```python
from build123d import *

# Parameters (mm, degrees)
F0_W     = 10
F0_H     = 20
F1_DEPTH = 10


with BuildPart() as f1:
    # F0 (on Front) → F1 (new body)
    with BuildSketch(Plane.XZ):
        with BuildLine():
            Line((-80.5, 20), (-203.5, 20))
            ThreePointArc((-203.5, 20), (-207.035534, 18.535534), (-208.5, 15))
            Line((-208.5, 15), (-208.5, 0))
            Line((-208.5, 0), (-158, 0))
            ThreePointArc((-158, 0), (-154.5, 3.5), (-151, 0))
            Line((-151, 0), (-80.5, 0))
            Line((-80.5, 0), (-80.5, 20))
        make_face()
        with Locations((-75.5, 10)):
            Rectangle(F0_W, F0_H)
        with BuildLine():
            Line((198.5, 20), (-70.5, 20))
            Line((-70.5, 20), (-70.5, 0))
            Line((-70.5, 0), (155, 0))
            ThreePointArc((155, 0), (158.5, 3.5), (162, 0))
            Line((162, 0), (198.5, 0))
            Line((198.5, 0), (198.5, 20))
        make_face()
        with BuildLine():
            Line((-80.5, -20), (-80.5, 0))
            Line((-80.5, 0), (-151, 0))
            ThreePointArc((-151, 0), (-154.5, -3.5), (-158, 0))
            Line((-158, 0), (-208.5, 0))
            Line((-208.5, 0), (-208.5, -15))
            ThreePointArc((-208.5, -15), (-207.035534, -18.535534), (-203.5, -20))
            Line((-203.5, -20), (-80.5, -20))
        make_face()
        with Locations((-75.5, -10)):
            Rectangle(F0_W, F0_H)
        with BuildLine():
            Line((203.5, 20), (198.5, 20))
            Line((198.5, 20), (198.5, 0))
            Line((198.5, 0), (208.5, 0))
            Line((208.5, 0), (208.5, 15))
            ThreePointArc((208.5, 15), (207.035534, 18.535534), (203.5, 20))
        make_face()
        with BuildLine():
            Line((155, 0), (-70.5, 0))
            Line((-70.5, 0), (-70.5, -20))
            Line((-70.5, -20), (198.5, -20))
            Line((198.5, -20), (198.5, 0))
            Line((198.5, 0), (162, 0))
            ThreePointArc((162, 0), (158.5, -3.5), (155, 0))
        make_face()
        with BuildLine():
            Line((208.5, 0), (198.5, 0))
            Line((198.5, 0), (198.5, -20))
            Line((198.5, -20), (203.5, -20))
            ThreePointArc((203.5, -20), (207.035534, -18.535534), (208.5, -15))
            Line((208.5, -15), (208.5, 0))
        make_face()
    extrude(amount=F1_DEPTH)


solid = f1.part
```
Work out the finished part from the listing and answer in its coordinate system (mm). Round coordinates to 2 decimals unless told otherwise and drop trailing zeros. Write each loop counter-clockwise with the first axis right and the second up, starting at its lowest first coordinate (ties: lowest second). Pieces come first, ordered by that corner, then holes.
1) Consider probe 1 along X at (y, z) = (-3, 0); probe 2 along Z at (x, y) = (-154.5, -2); probe 3 along X at (y, z) = (-7, 2). Determine where each line is inside the solid, lowest interval first.
2) A cutting plane is placed at B-B on z = 0. Determine the outline of the cut face in (x, y), and give its area (3 significant figures).
3) A cutting plane is placed at A-A on x = 158.5. Determine the outline of the cut face in (y, z), and give its area (3 significant figures).
4) Determine the mould class of faces 1 (the face through (-3, -5, -20)), 2 (the face through (208.5, -5, 0)), 3 (the face through (-151.16, -4.93, -1.05)) for opening direction Z: pulls with the +Z half, pulls with the -Z half, needs draft (parallel to the pull), parting line crosses it, or undercut.
Entries:
1. probe 1: x = -208.5 to -158, -151 to 155, 162 to 208.5
1. probe 2: z = -20 to -3.5, 3.5 to 20
1. probe 3: x = -208.5 to -157.37, -151.63 to 155.63, 161.37 to 208.5
2. outline: (-208.5, -10) - (-158, -10) - (-158, 0) - (-208.5, 0) - close; (-151, -10) - (155, -10) - (155, 0) - (-151, 0) - close; (162, -10) - (208.5, -10) - (208.5, 0) - (162, 0) - close
2. area: 4,030 mm2
3. outline: (-10, -20) - (0, -20) - (0, -3.5) - (-10, -3.5) - close; (-10, 3.5) - (0, 3.5) - (0, 20) - (-10, 20) - close
3. area: 330 mm2
4. face 1: pulls with the -Z half
4. face 2: needs draft
4. face 3: undercut
